Could you check a few things on this drawing? It's one solid part, dimensions in mm from its lowest x, y, z. A direction names the side the tool comes from. Give positions to 0.01 mm unless a question says otherwise; leave off trailing zeros. Loops run counter-clockwise (first coordinate to the right, second up) from the corner with the lowest first, then second, coordinate; pieces in that order, holes last. Notation, with made-up numbers: (31.25, 49.5) - (48.25, 49.5) arc R20 ccw to (48.25, 71.5) - close; hole circle Ø11 at (-31, 43). An arc over 180 degrees is marked (long way). Put each result on its own line as item: value. Start each with the question number.
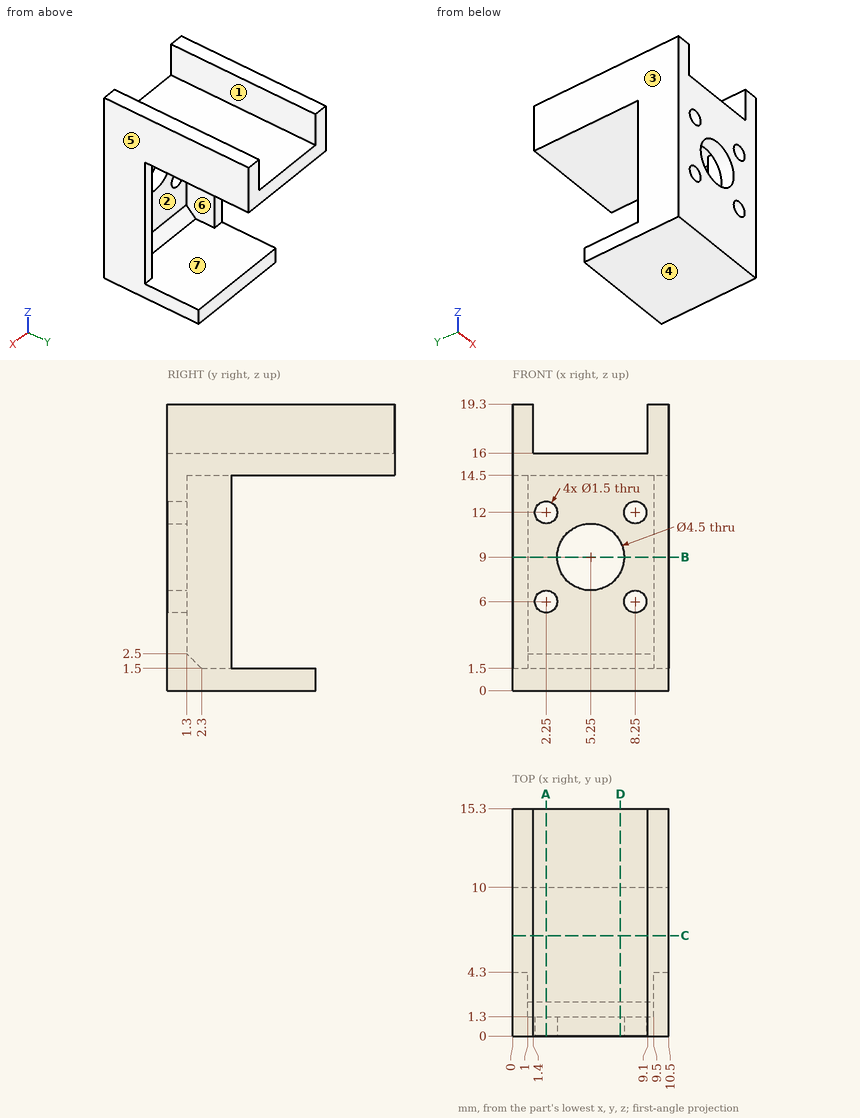
1) Thinking about a two-plate mould opening in X: for the marked faces 4, 5, 6 and 7, which applies, pulls with the +X half, pulls with the -X half, needs draft (parallel to the pull), parting line crosses it, or undercut?
2) Suppose I cut it at D-D on x = 7.25. Please give me the cut outline in (y, z).
3) Suppose I cut it at B-B on z = 9. Please give me the cut outline in (x, y).
4) Suppose I cut it at A-A on x = 2.25. Please give me the cut outline in (y, z).
5) I'm going to push flat-ended pins straight in: P1, Ø1.2, axis at x = 3.5, z = 1, coming from the +Y side; P2, Ø1.4, axis at x = 2.25, z = 12, coming from the -Y side; P3, Ø5, axis at x = 3, y = 10, coming from the -Z side; P4, Ø2, axis at x = 4, z = 8, coming from the +Y side. Where does each tip first touch, or does it pass through?
6) I need wall thicknesses on line 1 (X direction, y = 0.75, z = 6); line 2 (X direction, y = 0.4, z = 9); line 3 (X direction, y = 12.75, z = 16.75). Which ranges of each line are inside material? Lowest first, please.
7) Which directions (+Z, -Z, +X, -X, +Y, -Y) give clear straight access to the entire face, cutting with the end or side of a thin tool? Please do the marked faces 1, 2 and 3.
8) Suppose I cut it at C-C on y = 6.75. Please give me the cut outline in (x, z).
Ans:
1. face 4: needs draft
1. face 5: pulls with the +X half
1. face 6: undercut
1. face 7: undercut
2. outline: (0, 0) - (10, 0) - (10, 1.5) - (2.3, 1.5) - (1.3, 2.5) - (1.3, 7.97) - (0, 7.97) - close; (0, 10.03) - (1.3, 10.03) - (1.3, 14.5) - (15.3, 14.5) - (15.3, 16) - (0, 16) - close
3. outline: (0, 0) - (3, 0) - (3, 1.3) - (1, 1.3) - (1, 4.3) - (0, 4.3) - close; (7.5, 0) - (10.5, 0) - (10.5, 4.3) - (9.5, 4.3) - (9.5, 1.3) - (7.5, 1.3) - close
4. outline: (0, 0) - (10, 0) - (10, 1.5) - (2.3, 1.5) - (1.3, 2.5) - (1.3, 5.25) - (0, 5.25) - close; (0, 6.75) - (1.3, 6.75) - (1.3, 11.25) - (0, 11.25) - close; (0, 12.75) - (1.3, 12.75) - (1.3, 14.5) - (15.3, 14.5) - (15.3, 16) - (0, 16) - close
5. P1: stops at y = 10
5. P2: passes through
5. P3: stops at z = 0
5. P4: stops at y = 1.3
6. line 1: x = 0 to 1.5, 3 to 7.5, 9 to 10.5
6. line 2: x = 0 to 3, 7.5 to 10.5
6. line 3: x = 0 to 1.4, 9.1 to 10.5
7. face 1: +Z, +Y, -Y
7. face 2: +Y
7. face 3: +Z, -Z, -X, +Y, -Y
8. outline: (0, 0) - (10.5, 0) - (10.5, 1.5) - (0, 1.5) - close; (0, 14.5) - (10.5, 14.5) - (10.5, 19.3) - (9.1, 19.3) - (9.1, 16) - (1.4, 16) - (1.4, 19.3) - (0, 19.3) - close
